from build123d import *

# Parameters (mm, degrees)
SKETCH_1_W                  = 140
SKETCH_1_H                  = 160
EXTRUDE_1_DEPTH             = 6
SKETCH_3_W                  = 140
SKETCH_3_H                  = 4
SKETCH_3_H_2                = 3
EXTRUDE_3_DEPTH             = 94
CUT_EXTRUDE_1_DEPTH         = 190.73665961
SKETCH_5_W                  = 1.5
SKETCH_5_H                  = 153
CUT_EXTRUDE_2_DEPTH         = 1
HOLE_WIZARD_M21_D           = 3.5
HOLE_WIZARD_M21_DEPTH       = 3
CUT_EXTRUDE_3_REACH         = 203.246
SKETCH_9_R                  = 3
SKETCH_9_R_2                = 4.5
SKETCH_9_R_3                = 6
SKETCH_9_W                  = 50
SKETCH_9_H                  = 38
SKETCH_10_W                 = 54
SKETCH_10_H                 = 48
CUT_EXTRUDE_4_DEPTH         = 3
SKETCH_11_W                 = 2.5
SKETCH_11_H                 = 1.5
SKETCH_11_W_2               = 3
SKETCH_11_H_2               = 2
CUT_EXTRUDE_5_DEPTH         = 2.5
HOLE_WIZARD_M31_D           = 3.4
HOLE_WIZARD_M31_DEPTH       = 4
HOLE_WIZARD_M31_CBORE_D     = 6.5
HOLE_WIZARD_M31_CBORE_DEPTH = 2.4
CUT_EXTRUDE_6_REACH         = 203.246
SKETCH_15_W                 = 12.5
SKETCH_15_H                 = 19.2
SKETCH_15_W_2               = 27
SKETCH_15_H_2               = 20.5
HOLE_WIZARD_M22_D           = 2.2
HOLE_WIZARD_M22_DEPTH       = 1
HOLE_WIZARD_M23_D           = 3.5
HOLE_WIZARD_M23_DEPTH       = 3
CUT_EXTRUDE_7_REACH         = 202.056
SKETCH_24_W                 = 3
SKETCH_24_H                 = 1


with BuildPart() as part:
    # Эскиз1 → Бобышка-Вытянуть1 (new body)
    with BuildSketch(Plane(origin=(0, 0, 0), x_dir=(1, 0, 0), z_dir=(0, 1, 0))):
        Rectangle(SKETCH_1_W, SKETCH_1_H)
    extrude(amount=EXTRUDE_1_DEPTH)

    # Эскиз3 → Бобышка-Вытянуть3 (add)
    with BuildSketch(Plane(origin=(0, 6, 0), x_dir=(1, 0, 0), z_dir=(0, 1, 0))):
        with Locations((0, -78)):
            Rectangle(SKETCH_3_W, SKETCH_3_H)
        with Locations((0, 78.5)):
            Rectangle(SKETCH_3_W, SKETCH_3_H_2)
    extrude(amount=EXTRUDE_3_DEPTH)

    # Эскиз4 → Вырез-Вытянуть1 (cut, through all)
    with BuildSketch(Plane(origin=(70, 0, 0), x_dir=(0, 0, -1), z_dir=(1, 0, 0))):
        Polygon((80, 100), (80, 97), (78.5, 97), (78.5, 98), (77, 98), (77, 100), align=None)
    extrude(amount=-CUT_EXTRUDE_1_DEPTH, mode=Mode.SUBTRACT)

    # Эскиз5 → Вырез-Вытянуть2 (cut)
    with BuildSketch(Plane(origin=(0, 6, 0), x_dir=(1, 0, 0), z_dir=(0, 1, 0))):
        with Locations((67.75, 0.5)):
            Rectangle(SKETCH_5_W, SKETCH_5_H)
        with Locations((-67.75, 0.5)):
            Rectangle(SKETCH_5_W, SKETCH_5_H)
    extrude(amount=-CUT_EXTRUDE_2_DEPTH, mode=Mode.SUBTRACT)

    # Отверстие с зазором M21
    with Locations(Plane(origin=(0, 6, 0), x_dir=(1, 0, 0), z_dir=(0, 1, 0))):
        with Locations((-58.5, -25), (-38.5, -25), (-38.5, -50), (-58.5, -50), (-18.875, -25), (1.125, -25), (-18.875, -50), (1.125, -50), (21, -10), (21, -60), (58.5, -60), (58.5, -10), (-58.5, 57), (-58.5, 0), (58.5, 0), (58.5, 57)):
            Hole(HOLE_WIZARD_M21_D / 2, depth=HOLE_WIZARD_M21_DEPTH)

    # Эскиз9 → Вырез-Вытянуть3 (cut, up to next)
    with BuildSketch(Plane.XY.offset(80), mode=Mode.PRIVATE) as cut_extrude_3_sk1:
        with Locations((-25, 20)):
            Circle(SKETCH_9_R)
    cut_extrude_3_tool1 = extrude(cut_extrude_3_sk1.sketch, amount=-CUT_EXTRUDE_3_REACH, mode=Mode.PRIVATE) & part.part
    # Эскиз9 → Вырез-Вытянуть3 (cut, up to next)
    with BuildSketch(Plane.XY.offset(80), mode=Mode.PRIVATE) as cut_extrude_3_sk2:
        with Locations((0, 20)):
            Circle(SKETCH_9_R)
    cut_extrude_3_tool2 = extrude(cut_extrude_3_sk2.sketch, amount=-CUT_EXTRUDE_3_REACH, mode=Mode.PRIVATE) & part.part
    # Эскиз9 → Вырез-Вытянуть3 (cut, up to next)
    with BuildSketch(Plane.XY.offset(80), mode=Mode.PRIVATE) as cut_extrude_3_sk3:
        with Locations((25, 20)):
            Circle(SKETCH_9_R)
    cut_extrude_3_tool3 = extrude(cut_extrude_3_sk3.sketch, amount=-CUT_EXTRUDE_3_REACH, mode=Mode.PRIVATE) & part.part
    # Эскиз9 → Вырез-Вытянуть3 (cut, up to next)
    with BuildSketch(Plane.XY.offset(80), mode=Mode.PRIVATE) as cut_extrude_3_sk4:
        with Locations((50, 69)):
            Circle(SKETCH_9_R_2)
    cut_extrude_3_tool4 = extrude(cut_extrude_3_sk4.sketch, amount=-CUT_EXTRUDE_3_REACH, mode=Mode.PRIVATE) & part.part
    # Эскиз9 → Вырез-Вытянуть3 (cut, up to next)
    with BuildSketch(Plane.XY.offset(80), mode=Mode.PRIVATE) as cut_extrude_3_sk5:
        with Locations((50, 35)):
            Circle(SKETCH_9_R_3)
    cut_extrude_3_tool5 = extrude(cut_extrude_3_sk5.sketch, amount=-CUT_EXTRUDE_3_REACH, mode=Mode.PRIVATE) & part.part
    # Эскиз9 → Вырез-Вытянуть3 (cut, up to next)
    with BuildSketch(Plane.XY.offset(80), mode=Mode.PRIVATE) as cut_extrude_3_sk6:
        with Locations(Location((-50, 35, 0), (0, 0, 180))):
            Circle(SKETCH_9_R_3)
    cut_extrude_3_tool6 = extrude(cut_extrude_3_sk6.sketch, amount=-CUT_EXTRUDE_3_REACH, mode=Mode.PRIVATE) & part.part
    # Эскиз9 → Вырез-Вытянуть3 (cut, up to next)
    with BuildSketch(Plane.XY.offset(80), mode=Mode.PRIVATE) as cut_extrude_3_sk7:
        with Locations((0, 69)):
            Rectangle(SKETCH_9_W, SKETCH_9_H)
    cut_extrude_3_tool7 = extrude(cut_extrude_3_sk7.sketch, amount=-CUT_EXTRUDE_3_REACH, mode=Mode.PRIVATE) & part.part
    add(cut_extrude_3_tool1.solids().sort_by_distance((-25, 20, 80))[0], mode=Mode.SUBTRACT)
    add(cut_extrude_3_tool2.solids().sort_by_distance((0, 20, 80))[0], mode=Mode.SUBTRACT)
    add(cut_extrude_3_tool3.solids().sort_by_distance((25, 20, 80))[0], mode=Mode.SUBTRACT)
    add(cut_extrude_3_tool4.solids().sort_by_distance((50, 69, 80))[0], mode=Mode.SUBTRACT)
    add(cut_extrude_3_tool5.solids().sort_by_distance((50, 35, 80))[0], mode=Mode.SUBTRACT)
    add(cut_extrude_3_tool6.solids().sort_by_distance((-50, 35, 80))[0], mode=Mode.SUBTRACT)
    add(cut_extrude_3_tool7.solids().sort_by_distance((0, 69, 80))[0], mode=Mode.SUBTRACT)

    # Эскиз10 → Вырез-Вытянуть4 (cut)
    with BuildSketch(Plane(origin=(0, 0, 76), x_dir=(-1, 0, 0), z_dir=(0, 0, -1))):
        with Locations((2, 69)):
            Rectangle(SKETCH_10_W, SKETCH_10_H)
    extrude(amount=-CUT_EXTRUDE_4_DEPTH, mode=Mode.SUBTRACT)

    # Эскиз11 → Вырез-Вытянуть5 (cut)
    with BuildSketch(Plane(origin=(0, 0, 76), x_dir=(-1, 0, 0), z_dir=(0, 0, -1))):
        with Locations((0, 26.618347297)):
            Rectangle(SKETCH_11_W, SKETCH_11_H)
        with Locations((-25, 26.618347297)):
            Rectangle(SKETCH_11_W, SKETCH_11_H)
        with Locations((25, 26.618347297)):
            Rectangle(SKETCH_11_W, SKETCH_11_H)
        with Locations((-50, 78.5)):
            Rectangle(SKETCH_11_W_2, SKETCH_11_H_2)
    extrude(amount=-CUT_EXTRUDE_5_DEPTH, mode=Mode.SUBTRACT)

    # Цековка для винта с внутренним шестигранником с тонкой головкой M31
    with Locations(Plane.XY.offset(80)):
        with Locations((-65, 95), (65, 95)):
            CounterBoreHole(HOLE_WIZARD_M31_D / 2, HOLE_WIZARD_M31_CBORE_D / 2, HOLE_WIZARD_M31_CBORE_DEPTH, depth=HOLE_WIZARD_M31_DEPTH)

    # Эскиз15 → Вырез-Вытянуть6 (cut, up to next)
    with BuildSketch(Plane(origin=(0, 0, -80), x_dir=(-1, 0, 0), z_dir=(0, 0, -1)), mode=Mode.PRIVATE) as cut_extrude_6_sk1:
        with Locations((18.75, 30)):
            Rectangle(SKETCH_15_W, SKETCH_15_H)
    cut_extrude_6_tool1 = extrude(cut_extrude_6_sk1.sketch, amount=-CUT_EXTRUDE_6_REACH, mode=Mode.PRIVATE) & part.part
    # Эскиз15 → Вырез-Вытянуть6 (cut, up to next)
    with BuildSketch(Plane(origin=(0, 0, -80), x_dir=(-1, 0, 0), z_dir=(0, 0, -1)), mode=Mode.PRIVATE) as cut_extrude_6_sk2:
        with Locations((48.5, 30)):
            Rectangle(SKETCH_15_W_2, SKETCH_15_H_2)
    cut_extrude_6_tool2 = extrude(cut_extrude_6_sk2.sketch, amount=-CUT_EXTRUDE_6_REACH, mode=Mode.PRIVATE) & part.part
    add(cut_extrude_6_tool1.solids().sort_by_distance((-18.75, 30, -80))[0], mode=Mode.SUBTRACT)
    add(cut_extrude_6_tool2.solids().sort_by_distance((-48.5, 30, -80))[0], mode=Mode.SUBTRACT)

    # Отверстие с зазором M22
    with Locations(Plane(origin=(0, 3, 0), x_dir=(1, 0, 0), z_dir=(0, 1, 0))):
        with Locations((-58.5, -50), (-38.5, -50), (-18.875, -50), (1.125, -50), (1.125, -25), (-18.875, -25), (-38.5, -25), (-58.5, -25), (21, -10), (21, -60), (58.5, -60), (58.5, -10), (58.5, 0), (-58.5, 0), (58.5, 57), (-58.5, 57)):
            Hole(HOLE_WIZARD_M22_D / 2, depth=HOLE_WIZARD_M22_DEPTH)

    # Отверстие с зазором M23
    with Locations(Plane(origin=(0, 0, 76), x_dir=(-1, 0, 0), z_dir=(0, 0, -1))):
        with Locations((-28.9, 86), (-28.9, 51.75), (32.35, 86), (32.35, 51.75)):
            Hole(HOLE_WIZARD_M23_D / 2, depth=HOLE_WIZARD_M23_DEPTH)

    # Эскиз24 → Вырез-Вытянуть7 (cut, up to next)
    with BuildSketch(Plane(origin=(0, 0, -78.5), x_dir=(-1, 0, 0), z_dir=(0, 0, -1)), mode=Mode.PRIVATE) as cut_extrude_7_sk1:
        with Locations((-68.5, 97.5)):
            Rectangle(SKETCH_24_W, SKETCH_24_H)
    cut_extrude_7_tool1 = extrude(cut_extrude_7_sk1.sketch, amount=-CUT_EXTRUDE_7_REACH, mode=Mode.PRIVATE) & part.part
    # Эскиз24 → Вырез-Вытянуть7 (cut, up to next)
    with BuildSketch(Plane(origin=(0, 0, -78.5), x_dir=(-1, 0, 0), z_dir=(0, 0, -1)), mode=Mode.PRIVATE) as cut_extrude_7_sk2:
        with Locations((68.5, 97.5)):
            Rectangle(SKETCH_24_W, SKETCH_24_H)
    cut_extrude_7_tool2 = extrude(cut_extrude_7_sk2.sketch, amount=-CUT_EXTRUDE_7_REACH, mode=Mode.PRIVATE) & part.part
    add(cut_extrude_7_tool1.solids().sort_by_distance((68.5, 97.5, -78.5))[0], mode=Mode.SUBTRACT)
    add(cut_extrude_7_tool2.solids().sort_by_distance((-68.5, 97.5, -78.5))[0], mode=Mode.SUBTRACT)


solid = part.part
Could you check a few things on this model? Use its own coordinates, in mm. A direction names the side the tool comes from. Give positions to 0.01 mm unless a question says otherwise; leave off trailing zeros. Order: outer loops, then holes, each group sorted by start corner. A loop starts at its lowest first (then second) coordinate and runs counter-clockwise, first axis right, second up.
1. Thinking about a two-plate mould opening in Y: for faces 5 (the cylindrical face through (-0.65, 17.07, 78.03)), 6 (the flat face through (-70, 5, 24)), 7 (the flat face through (-1, 100, 78)), which applies, +Y half, -Y half, draft (parallel to the pull), parting line (faces both ways), or undercut?
Answers below:
face 5: undercut
face 6: draft
face 7: +Y half
2. Suppose I cut it at D-D (z = 30). Write out the boundary of the cut face in (x, y), plus the area to 3 significant figures.
Answers below:
outline: (-70, 0) - (70, 0) - (70, 6) - (68.5, 6) - (68.5, 5) - (67, 5) - (67, 6) - (-67, 6) - (-67, 5) - (-68.5, 5) - (-68.5, 6) - (-70, 6) - close
area: 837 mm2
3. Which directions (+Z, -Z, +X, -X, +Y, -Y) give clear straight access to the entire face, cutting with the end or side of a thin tool? Please do faces 1 (the flat face through (-1, 41, 76)), 2 (the cylindrical face through (-27.4, 18.2, 78)), 3 (the flat face through (-26, 71, 79)), 4 (the flat face through (-1, 48, -80)).
Answers below:
face 1: +X, -X, +Y
face 2: +Z
face 3: none
face 4: -Z, +X, -X, +Y, -Y
4. Suppose I cut it at A-A (x = 13). Write out the boundary of the cut face in (y, z), plus the area to 3 significant figures.
Answers below:
outline: (0, -80) - (97, -80) - (97, -78.5) - (98, -78.5) - (98, -77) - (6, -77) - (6, 76) - (45, 76) - (45, 79) - (50, 79) - (50, 80) - (0, 80) - close; (88, 79) - (93, 79) - (93, 76) - (100, 76) - (100, 80) - (88, 80) - close
area: 1,430 mm2
5. Suppose I cut it at B-B (y = 61.5). Write out the boundary of the cut face in (x, z).
Answers below:
outline: (-70, -80) - (70, -80) - (70, -77) - (-70, -77) - close; (-70, 76) - (-29, 76) - (-29, 79) - (-25, 79) - (-25, 80) - (-70, 80) - close; (25, 76) - (70, 76) - (70, 80) - (25, 80) - close
6. I need wall thicknesses on L1, parallel to Z at x = 21, y = 4.45; L2, parallel to Z at x = -58.5, y = 4.8; L3, parallel to Z at x = -38.5, y = 3.75. Which ranges of each line are inside material? Lowest first, please.
Answers below:
L1: z = -80 to 8.25, 11.75 to 58.25, 61.75 to 80
L2: z = -80 to -58.75, -55.25 to -1.75, 1.75 to 23.25, 26.75 to 48.25, 51.75 to 80
L3: z = -80 to 23.25, 26.75 to 48.25, 51.75 to 80
7. For pin 1 (1.5 mm diameter, centred on x = -19.5, z = -78, fed in from +Y); pin 2 (12 mm diameter, centred on x = -12, y = 58.5, fed in from +Z); pin 3 (0.8 mm diameter, centred on x = -69.5, z = 1, fed in from +Y), each with a flat end and sliding along its axis, tell me the tip position at first contact or that it passes through.
Answers below:
pin 1: stops at y = 98
pin 2: stops at z = -77
pin 3: stops at y = 6
8. Suppose I cut it at C-C (y = 9.5). Write out the boundary of the cut face in (x, z).
Answers below:
outline: (-70, -80) - (70, -80) - (70, -77) - (-70, -77) - close; (-70, 76) - (70, 76) - (70, 80) - (-70, 80) - close
